Build history of the part. All positions in model axes, mm. A direction names the side the tool comes from. Round coordinates to 2 decimals unless told otherwise and drop trailing zeros. Order: outer loops, then holes, each group sorted by start corner. A loop starts at its lowest first (then second) coordinate and runs counter-clockwise, first axis right, second up. Notation, with made-up numbers: M 7.25,68 L 51.25,68 A30 ccw 51.25,91 Z; hole C 62,82 d4. An arc over 180 degrees is marked long. One line per question, with ' | ' between items. Start each with the question number.
Autodesk Fusion 360 part; units mm, degrees
sketch "Sketch1" plane through (0, 0, 0) normal (0, 0, 1) x (1, 0, 0)
  line L0 (0, 0) -> (0, 40)
  line L1 (0, 40) -> (15, 40)
  line L2 (0, 0) -> (15, 0)
  arc A0 (15, 0) -> (15, 40) centre (0, 20) ccw
  line L3 (-6, -6) -> (16.8819, -6)
  arc A1 (16.8819, -6) -> (16.8819, 46) centre (0, 20) ccw
  line L4 (-6, 46) -> (16.8819, 46)
  line L5 (-6, -6) -> (-6, 46)
  dimension "d3" = 40
  dimension "d4" = 25
  dimension "d5" = 15
  dimension "d6" = -6
extrude "Extrude1" add sketch "Sketch1" along normal blind 5
chamfer "Chamfer1" distance 1.2 angle 45 4 faces at (18.0943, 45.1713, 3.3333) (1.6273, 46, 1.6667) (-6, 11.3333, 1.6667) (1.6273, -6, 1.6667)
chamfer "Chamfer2" distance 1 angle 45 4 faces at (5, 0, 1.6667) (0, 13.3333, 3.3333) (23.8152, 27.605, 3.3333) (5, 40, 1.6667)
Item 1: Cut at B-B on z = 2.95. Write the cut outline in (x, y).
Item 2: Wall check: line 1 along Y through (x, z) = (10, 2.65); line 2 along X through (y, z) = (20.5, 1.5) (3 decimals); line 3 along X through (y, z) = (29, 2.15). Give the ranges that are in metal, low to high. Write a range as [from, to].
Item 3: Two-plate mould, pull along X, no slides. Class faces 4 (the face through (7.4, 40.5, 4.5)), 5 (the face through (-2, 20, 0)), 6 (the face through (-5.18, -5.16, 4.26)): +X half, -X half, draft (parallel to the pull), parting line (faces both ways), or undercut.
Item 4: Tool access for faces 1 (the face through (0.5, 0.5, 2.5)), 2 (the face through (7.4, -0.5, 4.5)), 3 (the face through (5, -6, 2)): list every direction of +Z, -Z, +X, -X, +Y, -Y with a clear straight run to the whole face (end or side of a thin tool).
Item 5: Flat gauge pins, fed straight in: pin 1 (8 mm diameter, centred on x = 23, y = 6, fed in from -Z); pin 2 (3 mm diameter, centred on x = 25, z = 1, fed in from -Y); pin 3 (1.5 mm diameter, centred on y = 11, z = 3, fed in from +X). Where does each tip first touch, or does it go through?
Item 6: Cut at A-A on x = 7. Write the cut outline in (y, z), then the cut area to 3 significant figures.
Results found:
1) outline: M -6,-4.8 L -4.8,-6 L 15.68,-6 L 17.88,-5.33 A31 ccw 17.88,45.33 L 15.68,46 L -4.8,46 L -6,44.8 Z; hole M 0,1 L 1,0 L 14,0 L 15.79,0.62 A25 ccw 15.79,39.38 L 14,40 L 1,40 L 0,39 Z
2) line 1: y = [-6, 0], [40, 46] | line 2: x = [-6, 0], [24.995, 30.996] | line 3: x = [-6, 0], [23.32, 29.66]
3) face 4: undercut | face 5: draft | face 6: -X half
4) face 1: +Z, -Z | face 2: +Z | face 3: +Z, -Z, +X, -X, -Y
5) pin 1: stops at z = 0 | pin 2: stops at y = -0.2 | pin 3: stops at x = 29.88
6) outline: M -6,1.2 L -4.8,0 L -1,0 L 0,1 L 0,4 L -1,5 L -4.8,5 L -6,3.8 Z; M 40,1 L 41,0 L 44.8,0 L 46,1.2 L 46,3.8 L 44.8,5 L 41,5 L 40,4 Z | area: 55.1 mm^2
